```python
from build123d import *

# Parameters (mm, degrees)
SKETCH1_W           = 300
SKETCH1_H           = 350
BOSS_EXTRUDE1_DEPTH = 100
CUT_EXTRUDE1_DEPTH  = 362.42080737
FILLET1_R           = 10
SHELL1_START        = -130
SHELL1_DEPTH        = 260


# Read off the part's stored shape, not the designer's step: Shell1
with BuildPart() as part:
    # Sketch1 → Boss-Extrude1 (new body)
    with BuildSketch(Plane.XY):
        Rectangle(SKETCH1_W, SKETCH1_H)
    extrude(amount=BOSS_EXTRUDE1_DEPTH)

    # Sketch2 → Cut-Extrude1 (cut, through all)
    with BuildSketch(Plane.ZY.offset(150)):
        Polygon((0, -175), (100, -120), (100, -175), align=None)
    extrude(amount=-CUT_EXTRUDE1_DEPTH, mode=Mode.SUBTRACT)

    # Fillet1
    fillet1_edges = [part.edges().sort_by_distance(p)[0] for p in [
        (150, 27.5, 100),
        (150, -147.5, 50),
        (0, -120, 100),
        (-150, -147.5, 50),
        (0, 175, 100),
        (150, 0, 0),
        (0, -175, 0),
        (-150, 0, 0),
        (0, 175, 0),
        (150, 175, 50),
        (-150, 175, 50),
        (-150, 27.5, 100),
    ]]
    fillet(fillet1_edges, radius=FILLET1_R)

    # Shell1 outline → Shell1 (cut)
    with BuildSketch(Plane.YZ.offset(SHELL1_START)):
        Polygon((155, 20), (155, 100), (-97.174575579, 100), (-141.174575579, 20), align=None)
    extrude(amount=SHELL1_DEPTH, mode=Mode.SUBTRACT)


solid = part.part
```
Geometry check sheet. Reference: the model listing, model coordinates, mm. A direction names the side the tool comes from. Coordinates: 2 decimals unless noted, no trailing zeros. Order: outer loops, then holes, each group sorted by start corner. A loop starts at its lowest first (then second) coordinate and runs counter-clockwise, first axis right, second up. Notation, with made-up numbers: (84, -9.5) - (97, -9.5) arc R33 cw to (97, 20.5) - close; hole circle Ø7 at (40, -2.5). An arc over 180 degrees is marked (long way). Answer in a Markdown table with one row per item. Add a question column.
1. Section check C-C (y = 32). Enter the section's corners in (x, z), plus the area to 3 significant figures.
2. Material ranges on L1, parallel to X at y = 149.5, z = 21.5; L2, parallel to Z at x = -19.5, y = -13; L3, parallel to Z at x = 129.5, y = -118, recorded low to high. Write a range as [from, to].
3. Draft check along X on faces 1 (the face through (1.96, -166.62, 4.786)), 2 (the face through (-2, 155, 59)), 3 (the face through (-130, 5, 61)), 4 (the face through (146.993, -142.043, 54.005)). Enter one of: +X half, -X half, draft (parallel to the pull), parting line (faces both ways), or undercut.
4. Section check A-A (x = -91). Enter the section's corners in (y, z).
5. Access from +Z, -Z, +X, -X, +Y, -Y to the whole of each face (thin tool, end or side, straight path). Record for faces 5 (the face through (-1.82, -118.867, 60.56)), 6 (the face through (1.96, 172.15, 96.99)).
6. Section check B-B (y = -105.5). Enter the section's corners in (x, z), plus the area to 3 significant figures.
7. Gauge pin test, flat end, axial feed: pin 1 Ø12 at (x, y) = (-47.5, 131) entering from +Z. Record the tip position at first contact, or that the pin passes through.
Data:
| question | item | result |
|---|---|---|
| 1 | outline | (-150, 10) arc R10 ccw to (-140, 0) - (140, 0) arc R10 ccw to (150, 10) - (150, 90) arc R10 ccw to (140, 100) - (130, 100) - (130, 20) - (-130, 20) - (-130, 100) - (-140, 100) arc R10 ccw to (-150, 90) - close |
| 1 | area | 9,110 mm² |
| 2 | L1 | x = [-150, -130], [130, 150] |
| 2 | L2 | z = [0, 20] |
| 2 | L3 | z = [0, 20], [62.14, 99.2] |
| 3 | face 1 | draft |
| 3 | face 2 | undercut |
| 3 | face 3 | undercut |
| 3 | face 4 | +X half |
| 4 | outline | (-166.85, 14.82) arc R10 ccw to (-158.09, 0) - (165, 0) arc R10 ccw to (175, 10) - (175, 90) arc R10 ccw to (165, 100) - (155, 100) - (155, 20) - (-141.17, 20) - (-97.17, 100) - (-114.09, 100) arc R10 ccw to (-122.85, 94.82) - close |
| 5 | face 5 | none |
| 5 | face 6 | +Z, +X, -X, +Y |
| 6 | outline | (-150, 10) arc R10 ccw to (-140, 0) - (140, 0) arc R10 ccw to (150, 10) - (150, 90) arc R10 ccw to (140, 100) - (-140, 100) arc R10 ccw to (-150, 90) - close; hole (-130, 20) - (130, 20) - (130, 84.86) - (-130, 84.86) - close |
| 6 | area | 13,000 mm² |
| 7 | pin 1 | stops at z = 20 |
